Check sheet for the drawn part. Datum: minimum x, y, z corner. Units: mm. A direction names the side the tool comes from. Give positions to 0.01 mm unless a question says otherwise; leave off trailing zeros. Loops run counter-clockwise (first coordinate to the right, second up) from the corner with the lowest first, then second, coordinate; pieces in that order, holes last. Notation, with made-up numbers: (33.5, 48) - (53.5, 48) arc R14 ccw to (53.5, 57) - close; hole circle Ø5 at (63, 39.25). An arc over 180 degrees is marked (long way). Use one line per item in the form item = value.
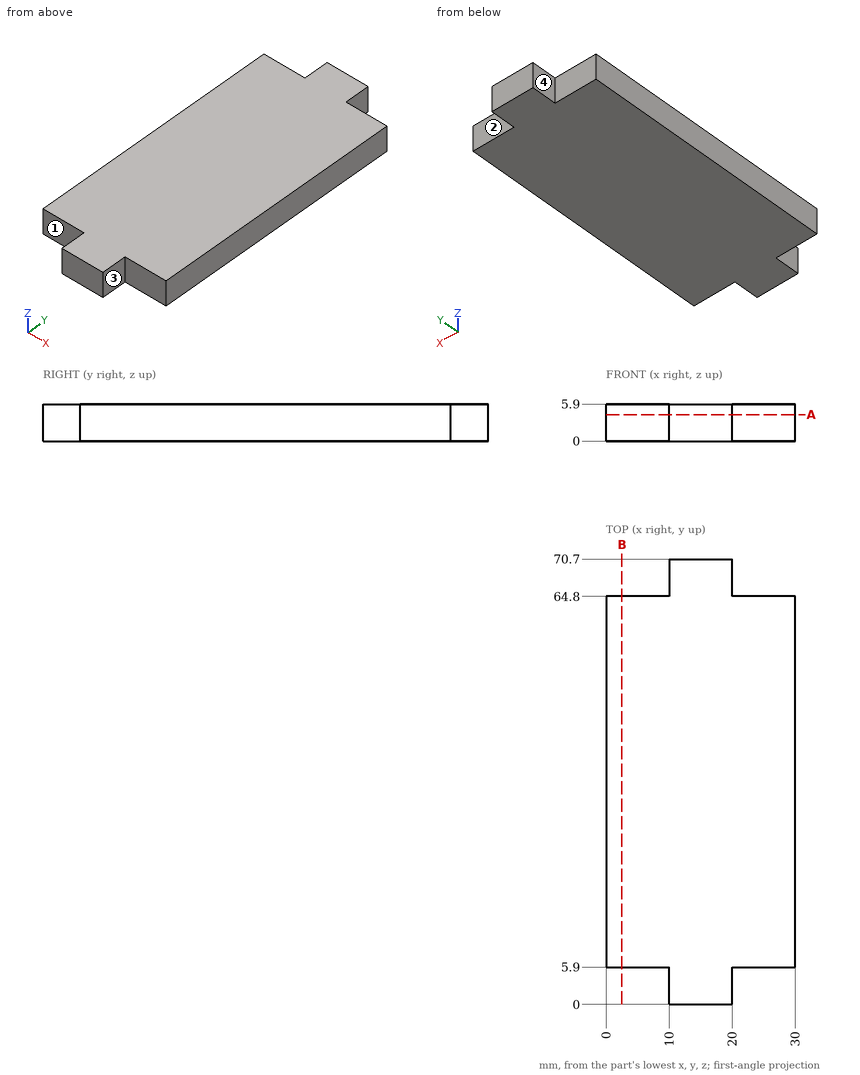
1. Scan lines: probe 1 along Y at (x, z) = (6.25, 2.5); probe 2 along X at (y, z) = (65.5, 0.95). Record each from-to range of solid material in increasing order.
Result set:
probe_1 = 5.9 to 64.8
probe_2 = 10 to 20
2. Depth check by flat-ended pin: pin 1 Ø10 at (x, y) = (23.5, 7.5) entering from -Z; pin 2 Ø3 at (x, z) = (6, 4) entering from -Y; pin 3 Ø1 at (x, z) = (4, 4.5) entering from +Y. Enter the tip coordinate at first touch or a pass-through.
Result set:
pin_1 = 0
pin_2 = 5.9
pin_3 = 64.8
3. Section check B-B, the plane x = 2.5. Record the cut outline in (y, z), then the cut area to 3 significant figures.
Result set:
outline = (5.9, 0) - (64.8, 0) - (64.8, 5.9) - (5.9, 5.9) - close
area = 348 mm²
4. Tool access check on the marked faces 1, 2, 3 and 4. Record the directions out of +Z, -Z, +X, -X, +Y, -Y that give a thin tool (end or side, any length) a straight path to the whole face; none if there is none.
Result set:
face_1 = +Z, -Z, -X, -Y
face_2 = +Z, -Z, +X, +Y
face_3 = +Z, -Z, +X, -Y
face_4 = +Z, -Z, -X, +Y
5. Section check A-A, the plane z = 4.2. Record the cut outline in (x, y), then the cut area to 4 significant figures.
Result set:
outline = (0, 5.9) - (10, 5.9) - (10, 0) - (20, 0) - (20, 5.9) - (30, 5.9) - (30, 64.8) - (20, 64.8) - (20, 70.7) - (10, 70.7) - (10, 64.8) - (0, 64.8) - close
area = 1,885 mm²
